```python
from build123d import *

# Parameters (mm, degrees)
DODANIE_WYCI_GNI_CIE2_DEPTH = 2
SZKIC4_R                    = 3
WYTNIJ_WYCI_GNI_CIE2_DEPTH  = 2
ZAOKR_GLENIE1_R             = 8
ZAOKR_GLENIE2_R             = 8


with BuildPart() as part:
    # Szkic3 → Dodanie-wyciągnięcie2 (new body)
    with BuildSketch(Plane.XY):
        with BuildLine():
            Line((1470.717856821, -27.5), (1500.717856821, -27.5))
            Line((1500.717856821, -27.5), (1500.717856821, -45.5))
            ThreePointArc((1500.717856821, -45.5), (1491.412577396, -46.218374962), (1483.717856821, -51.5))
            Line((1483.717856821, -51.5), (1470.717856821, -51.5))
            Line((1470.717856821, -51.5), (1470.717856821, -27.5))
        make_face()
    extrude(amount=DODANIE_WYCI_GNI_CIE2_DEPTH)

    # Szkic4 → Wytnij-wyciągnięcie2 (cut)
    with BuildSketch(Plane.XY.offset(2)):
        with Locations((1485.717856821, -33.5)):
            Circle(SZKIC4_R)
    extrude(amount=-WYTNIJ_WYCI_GNI_CIE2_DEPTH, mode=Mode.SUBTRACT)

    # Zaokrąglenie1
    zaokr_glenie1_edges = [part.edges().sort_by_distance(p)[0] for p in [
        (1470.717856821, -27.5, 1),
    ]]
    fillet(zaokr_glenie1_edges, radius=ZAOKR_GLENIE1_R)

    # Zaokrąglenie2
    zaokr_glenie2_edges = [part.edges().sort_by_distance(p)[0] for p in [
        (1500.717856821, -27.5, 1),
    ]]
    fillet(zaokr_glenie2_edges, radius=ZAOKR_GLENIE2_R)


solid = part.part
```
Work out the finished part from the listing and answer in its coordinate system (mm). Coordinates: 2 decimals unless noted, no trailing zeros. Loops run counter-clockwise (first coordinate to the right, second up) from the corner with the lowest first, then second, coordinate; pieces in that order, holes last.
1) A flat-ended cylindrical pin translates along its axis: pin 1 (1 mm diameter, centred on x = 1493.5, z = 1, fed in from +Y) (3 decimals). Find the tip coordinate at first contact, or state that the pin passes through.
Results:
pin 1: stops at y = -27.505
2) Section D-D (x = 1473.25) is taken. Give the vertices of the cut face in (y, z).
Results:
outline: (-51.5, 0) - (-29.66, 0) - (-29.66, 2) - (-51.5, 2) - close
3) For a pull along X with two mould halves and no side action, classify faces 1 (the flat face through (1500.718, -40, 1)), 2 (the cylindrical face through (1488.58, -32.6, 1.01)), 3 (the flat face through (1470.718, -44, 1)) as +X half, -X half, draft (parallel to the pull), parting line (faces both ways), or undercut.
Results:
face 1: +X half
face 2: undercut
face 3: -X half
4) Section C-C (y = -29.25) is taken. Give the vertices of the cut face in (x, z), plus the area to 3 significant figures.
Results:
outline: (1473.72, 0) - (1497.71, 0) - (1497.71, 2) - (1473.72, 2) - close
area: 48.0 mm2
5) Consider probe 1 along Y at (x, z) = (1486.25, 0.1); probe 2 along X at (y, z) = (-31.25, 0.5); probe 3 along Y at (x, z) = (1488.25, 1.65). Determine where each line is inside the solid, lowest interval first.
Results:
probe 1: y = -49.06 to -36.45, -30.55 to -27.5
probe 2: x = 1471.94 to 1483.73, 1487.7 to 1499.5
probe 3: y = -47.69 to -35.11, -31.89 to -27.5
6) Section B-B (y = -32) is taken. Give the vertices of the cut face in (x, z), plus the area to 3 significant figures.
Results:
outline: (1471.52, 0) - (1483.12, 0) - (1483.12, 2) - (1471.52, 2) - close; (1488.32, 0) - (1499.91, 0) - (1499.91, 2) - (1488.32, 2) - close
area: 46.4 mm2
7) Section A-A (z = 0.3) is taken. Give the vertices of the cut face in (x, y).
Results:
outline: (1470.72, -51.5) - (1483.72, -51.5) arc R18 cw to (1500.72, -45.5) - (1500.72, -35.5) arc R8 ccw to (1492.72, -27.5) - (1478.72, -27.5) arc R8 ccw to (1470.72, -35.5) - close; hole circle Ø6 at (1485.72, -33.5)
